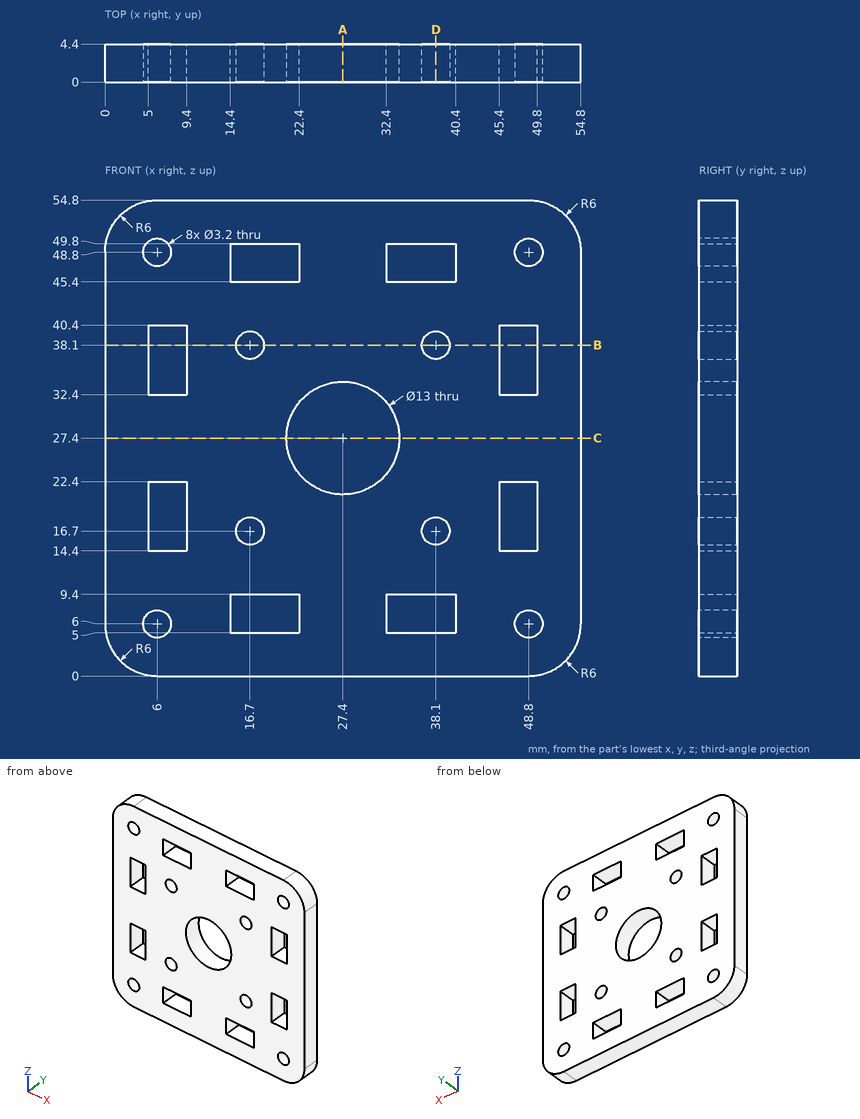
Study the drawing (mm; zero at the part's minimum x, y, z) and answer. Give positions to 0.01 mm unless a question says otherwise; leave off trailing zeros. Write each loop counter-clockwise with the first axis right and the second up, starting at its lowest first coordinate (ties: lowest second). Pieces come first, ordered by that corner, then holes. Notation, with made-up numbers: (-14, 72.5) -> (20, 72.5) arc R20 ccw to (20, 82.5) -> close; hole circle Ø1 at (24, -32.75). An arc over 180 degrees is marked (long way). Write item = value, one per line. Start each with the question number.
1) The part is cut by section A-A, the plane x = 27.4. Determine the outline of the cut face in (y, z), and give its area (3 significant figures).
2) The part is cut by section D-D, the plane x = 38.1. Determine the outline of the cut face in (y, z), and give its area (3 significant figures).
3) The part is cut by section B-B, the plane z = 38.1. Determine the outline of the cut face in (x, y).
4) Straight lines are drawn through the part: line 1 along Z through (x, y) = (16.7, 1.95); line 2 along Z through (x, y) = (9, 1); line 3 along X through (y, z) = (2.7, 48.8). For each, find the intervals that lie inside material, in ascending order.
5) The part is cut by section C-C, the plane z = 27.4. Determine the outline of the cut face in (x, y), and give its area (3 significant figures).
6) This flat-tipped pin is pushed along its axis until it touches: pin 1 (2 mm diameter, centred on x = 17.5, y = 3, fed in from -Z). Where does it stop, or does it pass through?
Solutions:
q1.outline = (0, 0) -> (4.4, 0) -> (4.4, 20.9) -> (0, 20.9) -> close; (0, 33.9) -> (4.4, 33.9) -> (4.4, 54.8) -> (0, 54.8) -> close
q1.area = 184 mm²
q2.outline = (0, 0) -> (4.4, 0) -> (4.4, 5) -> (0, 5) -> close; (0, 9.4) -> (4.4, 9.4) -> (4.4, 15.1) -> (0, 15.1) -> close; (0, 18.3) -> (4.4, 18.3) -> (4.4, 36.5) -> (0, 36.5) -> close; (0, 39.7) -> (4.4, 39.7) -> (4.4, 45.4) -> (0, 45.4) -> close; (0, 49.8) -> (4.4, 49.8) -> (4.4, 54.8) -> (0, 54.8) -> close
q2.area = 174 mm²
q3.outline = (0, 0) -> (5, 0) -> (5, 4.4) -> (0, 4.4) -> close; (9.4, 0) -> (15.1, 0) -> (15.1, 4.4) -> (9.4, 4.4) -> close; (18.3, 0) -> (36.5, 0) -> (36.5, 4.4) -> (18.3, 4.4) -> close; (39.7, 0) -> (45.4, 0) -> (45.4, 4.4) -> (39.7, 4.4) -> close; (49.8, 0) -> (54.8, 0) -> (54.8, 4.4) -> (49.8, 4.4) -> close
q4.line_1 = 0 to 5, 9.4 to 15.1, 18.3 to 36.5, 39.7 to 45.4, 49.8 to 54.8
q4.line_2 = 0 to 14.4, 22.4 to 32.4, 40.4 to 54.8
q4.line_3 = 0 to 4.4, 7.6 to 14.4, 22.4 to 32.4, 40.4 to 47.2, 50.4 to 54.8
q5.outline = (0, 0) -> (20.9, 0) -> (20.9, 4.4) -> (0, 4.4) -> close; (33.9, 0) -> (54.8, 0) -> (54.8, 4.4) -> (33.9, 4.4) -> close
q5.area = 184 mm²
q6.pin_1 = 0
